```python
from build123d import *

# Parameters (mm, degrees)
CUT_EXTRUDE1_DEPTH      = 41.98579449
CUT_EXTRUDE1_DEPTH_BACK = 41.98579449
SKETCH2_R               = 2.38125
CHAMFER1_SIZE           = 2.38125


with BuildPart() as part:
    # Sketch1 → Pin Body (revolve)
    with BuildSketch(Plane.XY, mode=Mode.PRIVATE) as pin_body_sk:
        Polygon((-34.29, 0), (-34.29, 15.875), (-27.94, 15.875), (-27.94, 9.525), (34.29, 9.525), (34.29, 0), align=None)
    revolve(pin_body_sk.sketch.rotate(Axis((-34.29, 0, 0), (1, 0, 0)), 90), axis=Axis((-34.29, 0, 0), (1, 0, 0)))

    # Sketch2 → Cut-Extrude1 (cut, two sides: drawn at the far end of the back side and taken through both)
    with BuildSketch(Plane.XY.offset(-CUT_EXTRUDE1_DEPTH_BACK)):
        with Locations((27.94, 0)):
            Circle(SKETCH2_R)
    extrude(amount=CUT_EXTRUDE1_DEPTH + CUT_EXTRUDE1_DEPTH_BACK, mode=Mode.SUBTRACT)

    # Chamfer1
    chamfer1_edges = [part.edges().sort_by_distance(p)[0] for p in [
        (34.29, 0, -9.525),
    ]]
    chamfer(chamfer1_edges, length=CHAMFER1_SIZE)


solid = part.part
```
CAD build for the part. Positions are in the model's coordinates, mm. A direction names the side the tool comes from. Round coordinates to 2 decimals unless told otherwise and drop trailing zeros. Loops run counter-clockwise (first coordinate to the right, second up) from the corner with the lowest first, then second, coordinate; pieces in that order, holes last. Notation, with made-up numbers: M 61.5,-21 L 75.5,-21 A3 ccw 75.5,-17 Z; hole C -18,-16.75 d4. An arc over 180 degrees is marked long. Use a Markdown table: item, result. Add a question column.
(1) Cut at C-C (x = 27.94). Give the cut face in (y, z) (3 decimals), and give its area (3 significant figures).
(2) Cut at B-B (y = 0). Give the cut face in (x, z) (3 decimals).
(3) Drill centre lines: line 1 (X direction, y = 0, z = -2.5); line 2 (X direction, y = 14, z = 7); line 3 (X direction, y = -1.5, z = -1). Where is each one in solid material? Low to high.
(4) Cut at D-D (x = 18). Give the cut face in (y, z) (3 decimals), and give its area (3 significant figures).
(5) Flat gauge pins, fed straight in: pin 1 (5.5 mm diameter, centred on x = 27.94, y = 0, fed in from +Z) (3 decimals); pin 2 (5 mm diameter, centred on x = 6, y = -9.5, fed in from -Z); pin 3 (3 mm diameter, centred on x = 20, y = -4.5, fed in from +Z). Where does each tip first touch, or does it go through?
(6) Which spindle directions (+Z, -Z, +X, -X, +Y, -Y) get a long thin tool onto all of the face, cutting with end or side? Do faces 4 (the face through (2.403, -2.861, 9.085)), 5 (the face through (-34.29, 0, 0)). Say none if no direction does.
(7) Cut at A-A (z = 0). Give the cut face in (x, y) (1 decimal), and give its area (3 significant figures).
(8) Pull direction Y, two halves, no side cores. Call faces 1 (the face through (-31.071, 15.497, -3.441)), 2 (the face through (25.56, 0.1, -0.13)), 3 (the face through (34.29, 0, 0)): +Y half, -Y half, draft (parallel to the pull), parting line (faces both ways), or undercut.
Geometry says:
| question | item | result |
|---|---|---|
| 1 | outline | M -2.381,-9.223 L -2.381,9.223 A9.525 ccw Z; M 2.381,-9.223 A9.525 ccw 2.381,9.223 Z |
| 1 | area | 195 mm² |
| 2 | outline | M -34.29,-15.875 L -27.94,-15.875 L -27.94,-9.525 L 25.559,-9.525 L 25.559,9.525 L -27.94,9.525 L -27.94,15.875 L -34.29,15.875 Z; M 30.321,-9.525 L 31.909,-9.525 L 34.29,-7.144 L 34.29,7.144 L 31.909,9.525 L 30.321,9.525 Z |
| 3 | line 1 | x = -34.29 to 25.56, 30.32 to 34.29 |
| 3 | line 2 | x = -34.29 to -27.94 |
| 3 | line 3 | x = -34.29 to 26.09, 29.79 to 34.29 |
| 4 | outline | C 0,0 d19.05 |
| 4 | area | 285 mm² |
| 5 | pin 1 | stops at z = 9.525 |
| 5 | pin 2 | stops at z = -6.46 |
| 5 | pin 3 | stops at z = 9.04 |
| 6 | face 4 | +X |
| 6 | face 5 | +Z, -Z, -X, +Y, -Y |
| 7 | outline | M -34.3,-15.9 L -27.9,-15.9 L -27.9,-9.5 L 31.9,-9.5 L 34.3,-7.1 L 34.3,7.1 L 31.9,9.5 L -27.9,9.5 L -27.9,15.9 L -34.3,15.9 Z; hole C 27.9,0 d4.8 |
| 7 | area | 1,360 mm² |
| 8 | face 1 | parting line |
| 8 | face 2 | undercut |
| 8 | face 3 | draft |
